Model file for the job. Use its own axes, mm. Face numbers are marked on the shaded views. Give positions to 0.01 mm unless a question says otherwise; leave off trailing zeros. Loops run counter-clockwise (first coordinate to the right, second up) from the corner with the lowest first, then second, coordinate; pieces in that order, holes last. Notation, with made-up numbers: M 45,77 L 81,77 A34 cw 81,108 Z; hole C 71.25,60 d10. An arc over 180 degrees is marked long. Answer in a Markdown table with one row per item.
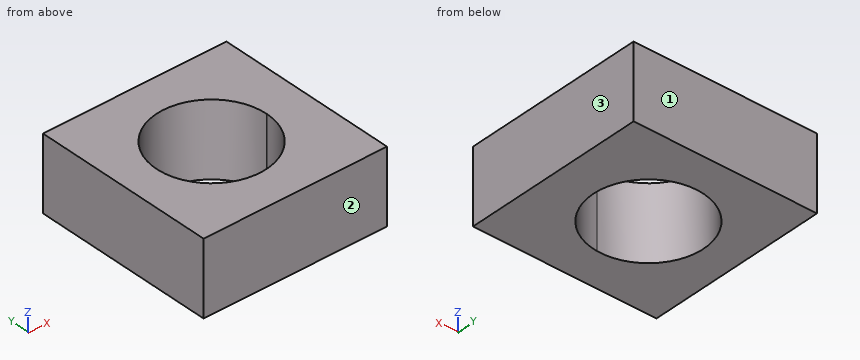
```python
from build123d import *

# Parameters (mm, degrees)
F1_DEPTH = 10


with BuildPart() as f1:
    # F0 (on Top) → F1 (new body)
    with BuildSketch(Plane.XY):
        with BuildLine():
            Line((-69.7358559817, 12.4485804441), (-94.7358559817, 12.4485804441))
            Line((-94.7358559817, 12.4485804441), (-94.7358559817, -12.5514195559))
            Line((-94.7358559817, -12.5514195559), (-82.2358559817, -12.5514195559))
            Line((-82.2358559817, -12.5514195559), (-82.2358559817, -7.4881173271))
            ThreePointArc((-82.2358559817, -7.4881173271), (-88.1083383981, 5.1519349585), (-75.1578736305, 0))
            ThreePointArc((-75.1578736305, 0), (-75.1579176973, -0.025709929), (-75.1580498973, -0.0514195559))
            Line((-75.1580498973, -0.0514195559), (-69.7358559817, -0.0514195559))
            Line((-69.7358559817, -0.0514195559), (-69.7358559817, 12.4485804441))
        make_face()
        with BuildLine():
            Line((-69.7358559817, -12.5514195559), (-69.7358559817, -0.0514195559))
            Line((-69.7358559817, -0.0514195559), (-75.1580498973, -0.0514195559))
            ThreePointArc((-75.1580498973, -0.0514195559), (-77.2251016718, -5.1705888296), (-82.2358559817, -7.4881173271))
            Line((-82.2358559817, -7.4881173271), (-82.2358559817, -12.5514195559))
            Line((-82.2358559817, -12.5514195559), (-69.7358559817, -12.5514195559))
        make_face()
    extrude(amount=F1_DEPTH)


solid = f1.part
```
Q1. Saw through at B-B (x = -89.5). Give the cut face in (y, z).
Reported:
| item | result |
|---|---|
| outline | M -12.55,0 L -3.07,0 L -3.07,10 L -12.55,10 Z; M 3.07,0 L 12.45,0 L 12.45,10 L 3.07,10 Z |
Q2. Mould opens along Y. For the marked faces 1, 2 and 3 say: released by +Y, released by -Y, zero draft, split by the parting line, or undercut.
Reported:
| item | result |
|---|---|
| face 1 | released by +Y |
| face 2 | released by -Y |
| face 3 | zero draft |
Q3. Probe probe 1 along X at (y, z) = (0, 4.25); probe 2 along Y at (x, z) = (-83, 8); probe 3 along Y at (x, z) = (-89.25, 4.75). List the from-to ranges inside material, lowest first.
Reported:
| item | result |
|---|---|
| probe 1 | -94.74 to -90.16, -75.16 to -69.74 |
| probe 2 | -12.55 to -7.49, 7.49 to 12.45 |
| probe 3 | -12.55 to -3.58, 3.58 to 12.45 |
Q4. Saw through at C-C (y = 1). Give the cut face in (x, z).
Reported:
| item | result |
|---|---|
| outline | M -94.74,0 L -90.09,0 L -90.09,10 L -94.74,10 Z; M -75.22,0 L -69.74,0 L -69.74,10 L -75.22,10 Z |
Q5. Saw through at A-A (z = 5). Give the cut face in (x, y), and give its area (3 significant figures).
Reported:
| item | result |
|---|---|
| outline | M -94.74,-12.55 L -69.74,-12.55 L -69.74,12.45 L -94.74,12.45 Z; hole M -75.16,-0.05 A7.5 ccw -75.16,0 A7.5 ccw long Z |
| area | 448 mm² |
